from build123d import *

# Parameters (mm, degrees)
SKETCH2_R           = 3.81
BOSS_EXTRUDE1_DEPTH = 3.175
SKETCH3_R           = 1.4605
CUT_EXTRUDE1_DEPTH  = 3.175


with BuildPart() as part:
    # Sketch2 → Boss-Extrude1 (new body)
    with BuildSketch(Plane.XY):
        with Locations((193.674999999, 14.287500001)):
            Circle(SKETCH2_R)
        Polygon((192.86290311, 18.009945251), (194.487096888, 10.56505475), (241.287043978, 20.775034718), (239.6628502, 28.219925218), align=None)
    extrude(amount=BOSS_EXTRUDE1_DEPTH)

    # Sketch3 → Cut-Extrude1 (cut)
    with BuildSketch(Plane.XY.offset(3.175)):
        with Locations((193.674999999, 14.287500001)):
            Circle(SKETCH3_R)
    extrude(amount=-CUT_EXTRUDE1_DEPTH, mode=Mode.SUBTRACT)


solid = part.part
Design review of the part built by this model. Coordinates are the model's own, in mm. Coordinates: 2 decimals unless noted, no trailing zeros. Write each loop counter-clockwise with the first axis right and the second up, starting at its lowest first coordinate (ties: lowest second). Pieces come first, ordered by that corner, then holes. Notation, with made-up numbers: (-39.75, -2.75) - (1.25, -2.75) arc R21 ccw to (1.25, 17.25) - close; hole circle Ø7 at (50.25, 43). An arc over 180 degrees is marked (long way). Use one line per item in the form item = value.
Q1. Consider section B-B (z = 2.15). Write out the cut boundary in (x, y) (1 decimal), plus the area to 3 significant figures.
Taken from the geometry:
outline = (192.9, 18) arc R3.8 ccw to (194.5, 10.6) - (241.3, 20.8) - (239.7, 28.2) - close; hole circle Ø2.9 at (193.7, 14.3)
area = 381 mm^2
Q2. Consider section D-D (y = 24.25). Write out the cut boundary in (x, z) (3 decimals), plus the area to 3 significant figures.
Taken from the geometry:
outline = (221.466, 0) - (240.529, 0) - (240.529, 3.175) - (221.466, 3.175) - close
area = 60.5 mm^2
Q3. Consider section A-A (y = 13.5). Write out the cut boundary in (x, z) (3 decimals).
Taken from the geometry:
outline = (189.947, 0) - (192.445, 0) - (192.445, 3.175) - (189.947, 3.175) - close; (194.905, 0) - (207.94, 0) - (207.94, 3.175) - (194.905, 3.175) - close
Q4. Consider section C-C (x = 206). Write out the cut boundary in (y, z) (3 decimals), plus the area to 3 significant figures.
Taken from the geometry:
outline = (13.077, 0) - (20.876, 0) - (20.876, 3.175) - (13.077, 3.175) - close
area = 24.8 mm^2
Q5. Insertion check: pin 1 Ø1.5 at (y, z) = (24.5, 1) entering from +X; pin 2 Ø2.5 at (x, y) = (193.67, 14.29) entering from -Z. Each pin has a flat end and moves straight along its axis. Give the tip position at first contact, or say it passes through.
Taken from the geometry:
pin_1 = 240.64
pin_2 = through
Q6. For probe 1 along Y at (x, z) = (210.5, 0.5); probe 2 along Y at (x, z) = (235, 0.95), list the stretches that pass through material, from the lowest coordinate up.
Taken from the geometry:
probe_1 = 14.06 to 21.86
probe_2 = 19.4 to 27.2
Q7. The part is to be moulded in two halves that separate along Y. For faces 1 (the flat face through (215, 19, 0)), 2 (the cylindrical face through (189.936, 13.557, 1.565)), 3 (the cylindrical face through (192.216, 14.352, 1.61)), 4 (the flat face through (216.59, 23.186, 1.565)), say which applies: +Y half, -Y half, draft (parallel to the pull), parting line (faces both ways), or undercut.
Taken from the geometry:
face_1 = draft
face_2 = parting line
face_3 = undercut
face_4 = +Y half
